For this review, take the finished solid that the model builds, in its own axes (mm). Face numbers are marked on the shaded views. A direction names the side the tool comes from. Give positions to 0.01 mm unless a question says otherwise; leave off trailing zeros. Order: outer loops, then holes, each group sorted by start corner. A loop starts at its lowest first (then second) coordinate and runs counter-clockwise, first axis right, second up. Notation, with made-up numbers: M -10.5,14 L 30.5,14 A17 ccw 30.5,36 Z; hole C 44.5,-31.75 d11. An arc over 180 degrees is marked long. Answer as CSV lines item,"result". Start each with the question number.
1. Machinability: for the marked faces 4, 5, 6 and 7, which of the approach directions +Z, -Z, +X, -X, +Y, -Y give a long, thin tool a straight path to every point of the face, cutting with its end or side? Answer none if there is none.
2. Mouldability with a two-part tool opening along X and no side actions: class the marked faces 1, 2 and 3 as pulls with the +X half, pulls with the -X half, needs draft (parallel to the pull), parting line crosses it, or undercut.
3. We need section A-A, the plane x = 82. Give the boundary of the cut face in (y, z) (3 decimals), and give its area (3 significant figures).
4. We need section D-D, the plane y = -14. Give the boundary of the cut face in (x, z) (3 decimals).
5. We need section B-B, the plane y = 52. Give the boundary of the cut face in (x, z) (3 decimals).
6. We need section C-C, the plane z = -0.5. Give the boundary of the cut face in (x, y) (3 decimals).
7. Clearance check with flat-ended pins moving along their axes: P1, Ø16.5, axis at x = 14.5, y = -44.5, coming from the +Z side (3 decimals); P2, Ø15, axis at x = 97, y = -12, coming from the -Z side; P3, Ø8, axis at y = 14.5, z = 21, coming from the +X side (3 decimals); P4, Ø5, axis at x = 6.5, z = 52, coming from the -Y side. State where each tip first meets the part, or that it passes through.
8. For line 1 along Z through (x, y) = (-11, 39.5) (3 decimals); line 2 along Z through (x, y) = (56, 24); line 3 along X through (y, z) = (10, 26.5) (3 decimals), list the stretches that pass through material, from the lowest coordinate up.
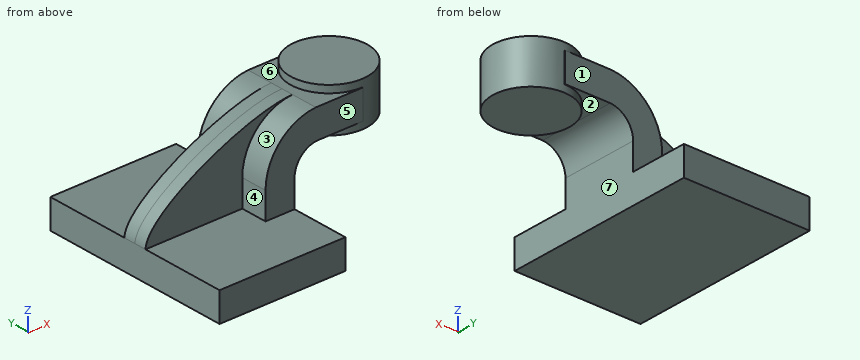
from build123d import *

# Parameters (mm, degrees)
F1_DEPTH = 63.5
F0_W     = 25.7461559653
F0_H     = 19.0207560397
F2_DEPTH = 25.4
F3_DEPTH = 7.9375


# Not quite as in the source:
# - a feature names something its author has since deleted; it is built from what else it names


with BuildPart() as f1:
    # F0 (on Front) → F1 (new body, symmetric)
    with BuildSketch(Plane.XZ):
        Polygon((22.225, 9.525), (-41.275, 9.525), (-41.275, -9.525), (41.275, -9.525), (41.275, 9.525), align=None)
    extrude(amount=F1_DEPTH, both=True)

    # F0 (on Front) → F2 (join, symmetric)
    with BuildSketch(Plane.XZ):
        with BuildLine():
            Line((22.225, 27.0245699669), (22.225, 9.525))
            Line((22.225, 9.525), (41.275, 9.525))
            Line((41.275, 9.525), (41.275, 27.0245699669))
            ThreePointArc((41.275, 27.0245699669), (45.6179930488, 37.9345855799), (56.2707090616, 42.8752))
            Line((56.2707090616, 42.8752), (60.325, 42.8752))
            Line((60.325, 42.8752), (60.325, 61.8959560397))
            Line((60.325, 61.8959560397), (55.2155599356, 61.8959560397))
            ThreePointArc((55.2155599356, 61.8959560397), (31.7795847073, 51.0266043156), (22.225, 27.0245699669))
        make_face()
        with Locations((73.1980779827, 52.3855780199)):
            Rectangle(F0_W, F0_H)
    extrude(amount=F2_DEPTH, both=True)

    # F0 (on Front) → F3 (join, symmetric)
    with BuildSketch(Plane.XZ):
        with BuildLine():
            add(Edge.make_bspline(
                [(-41.275, 9.525), (-40.530513972, 29.3039940298), (25.5654975772, 61.4196136594), (55.2155599356, 61.8959560397)],
                knots=[0, 0, 0, 0, 109.7868170282, 109.7868170282, 109.7868170282, 109.7868170282], degree=3))
            Line((-41.275, 9.525), (22.225, 9.525))
            Line((22.225, 9.525), (22.225, 27.0245699669))
            ThreePointArc((22.225, 27.0245699669), (31.7795847073, 51.0266043156), (55.2155599356, 61.8959560397))
        make_face()
    extrude(amount=F3_DEPTH, both=True)

    # F0 (on Front) → F4 (revolve)
    with BuildSketch(Plane.XZ):
        Polygon((86.0711559653, 66.675), (86.0711559653, 61.8959560397), (86.0711559653, 42.8752), (86.0711559653, 38.1), (111.125, 38.1), (111.125, 66.675), align=None)
    revolve(axis=Axis((86.0711559653, 0, 52.3875), (0, 0, 1)))


solid = f1.part
Result set:
1,face 4,"+Z, -X, -Y"
1,face 5,"+Z, +X, -X, -Y"
1,face 6,"+Z, -X"
1,face 7,"-Z, +X, +Y, -Y"
2,face 1,"needs draft"
2,face 2,"undercut"
2,face 3,"pulls with the -X half"
3,outline,"M -25.4,42.875 L -24.721,42.875 L -24.721,38.1 L 24.721,38.1 L 24.721,42.875 L 25.4,42.875 L 25.4,61.896 L 24.721,61.896 L 24.721,66.675 L -24.721,66.675 L -24.721,61.896 L -25.4,61.896 Z"
3,area,"1,440 mm2"
4,outline,"M -41.275,-9.525 L 41.275,-9.525 L 41.275,27.025 A15.875 cw 56.271,42.875 L 65.294,42.875 L 65.294,38.1 L 106.848,38.1 L 106.848,66.675 L 65.294,66.675 L 65.294,61.896 L 55.216,61.896 A34.925 ccw 22.225,27.025 L 22.225,9.525 L -41.275,9.525 Z"
5,outline,"M -41.275,-9.525 L 41.275,-9.525 L 41.275,9.525 L -41.275,9.525 Z"
6,outline,"M -41.275,-63.5 L 41.275,-63.5 L 41.275,63.5 L -41.275,63.5 Z"
7,P1,"z = 9.525"
7,P2,"z = 38.1"
7,P3,"x = 41.275"
7,P4,"through"
8,line 1,"-9.525 to 9.525"
8,line 2,"42.86 to 61.9"
8,line 3,"22.225 to 41.275"
